```python
from build123d import *

# Parameters (mm, degrees)
SKETCH_1_W          = 60
SKETCH_1_H          = 10
EXTRUDE_1_DEPTH     = 10
SKETCH_3_R          = 1.4
CUT_EXTRUDE_1_DEPTH = 20


with BuildPart() as part:
    # 草图1 → 凸台-拉伸1 (new body)
    with BuildSketch(Plane(origin=(0, 0, 0), x_dir=(1, 0, 0), z_dir=(0, 1, 0))):
        with Locations((30, 5)):
            Rectangle(SKETCH_1_W, SKETCH_1_H)
    extrude(amount=EXTRUDE_1_DEPTH)

    # 草图3 → 切除-拉伸1 (cut)
    with BuildSketch(Plane.XY):
        with Locations((6, 5)):
            Circle(SKETCH_3_R)
        with Locations((54, 5)):
            Circle(SKETCH_3_R)
    extrude(amount=-CUT_EXTRUDE_1_DEPTH, mode=Mode.SUBTRACT)


solid = part.part
```
Model file for the job. Use its own axes, mm. Coordinates: 2 decimals unless noted, no trailing zeros. Order: outer loops, then holes, each group sorted by start corner. A loop starts at its lowest first (then second) coordinate and runs counter-clockwise, first axis right, second up. Notation, with made-up numbers: (42.25, 76.25) -> (61.25, 76.25) arc R24 cw to (61.25, 98.25) -> close; hole circle Ø11 at (38.5, 53). An arc over 180 degrees is marked (long way). Answer as a JSON object with one key per item and string values. Group by question number.
1) Drill centre lines: L1, parallel to Y at x = 6, z = -3.5; L2, parallel to X at y = 5.5, z = -6.5; L3, parallel to Y at x = 6.5, z = -5.5. Where is each one in solid material? Low to high.
2) Cut at B-B, the plane z = -4.5. Write the cut outline in (x, y).
3) Pull direction Y, two halves, no side cores. Call faces 1 (the face through (30, 5, -10)), 2 (the face through (55.335, 5.421, -4.93)), 3 (the face through (30, 10, -5)): +Y half, -Y half, draft (parallel to the pull), parting line (faces both ways), or undercut.
4) Cut at A-A, the plane x = 54. Write the cut outline in (y, z), then the cut area to 3 significant figures.
5) Flat gauge pin, fed straight in: pin 1 (1.7 mm diameter, centred on x = 6, y = 5, fed in from +Z). Where does the tip first touch, or does it go through?
Check values:
{
 "1": {"L1": "y = 0 to 3.6, 6.4 to 10", "L2": "x = 0 to 4.69, 7.31 to 52.69, 55.31 to 60", "L3": "y = 0 to 3.69, 6.31 to 10"},
 "2": {"outline": "(0, 0) -> (60, 0) -> (60, 10) -> (0, 10) -> close; hole circle Ø2.8 at (6, 5); hole circle Ø2.8 at (54, 5)"},
 "3": {"face 1": "draft", "face 2": "undercut", "face 3": "+Y half"},
 "4": {"outline": "(0, -10) -> (3.6, -10) -> (3.6, 0) -> (0, 0) -> close; (6.4, -10) -> (10, -10) -> (10, 0) -> (6.4, 0) -> close", "area": "72.0 mm²"},
 "5": {"pin 1": "passes through"}
}
